from build123d import *

# Parameters (mm, degrees)
BOSS_EXTRUDE1_DEPTH     = 34
SKETCH2_R               = 35
BOSS_EXTRUDE2_DEPTH     = 10
SKETCH3_R               = 25
BOSS_EXTRUDE3_DEPTH     = 80
CUT_EXTRUDE2_START      = -40
CUT_EXTRUDE2_DEPTH      = 40
CUT_EXTRUDE5_DEPTH      = 114.247516529
CUT_EXTRUDE5_DEPTH_BACK = 114.247516529
SKETCH11_W              = 43
SKETCH11_H              = 18


with BuildPart() as part:
    # Sketch1 → Boss-Extrude1 (new body)
    with BuildSketch(Plane(origin=(0, 0, 0), x_dir=(1, 0, 0), z_dir=(0, 1, 0))):
        Polygon((50, 0), (-50, 0), (-50, 10), (-32.679491924, 40), (32.679491924, 40), (50, 10), align=None)
    extrude(amount=BOSS_EXTRUDE1_DEPTH)

    # Sketch2 → Boss-Extrude2 (add)
    with BuildSketch(Plane.XY):
        with Locations((0, 17)):
            Circle(SKETCH2_R)
    extrude(amount=-BOSS_EXTRUDE2_DEPTH)

    # Sketch3 → Boss-Extrude3 (add)
    with BuildSketch(Plane.XY):
        with Locations((0, 17)):
            Circle(SKETCH3_R)
    extrude(amount=-BOSS_EXTRUDE3_DEPTH)

    # Sketch5 → Cut-Extrude2 (cut)
    with BuildSketch(Plane(origin=(0, 0, -80), x_dir=(-1, 0, 0), z_dir=(0, 0, -1)).offset(CUT_EXTRUDE2_START)):
        with BuildLine():
            ThreePointArc((-25, 17.00000011), (-21.213203465, 3.771243492), (-11, -5.449944321))
            Line((-11, -5.449944321), (-11, 39.449944321))
            ThreePointArc((-11, 39.449944321), (-21.213203406, 30.228756602), (-25, 17.00000011))
        make_face()
        with BuildLine():
            ThreePointArc((-25, 17.00000011), (-21.213203406, 30.228756602), (-11, 39.449944321))
            Line((-11, 39.449944321), (-11, 52))
            Line((-11, 52), (-25, 52))
            Line((-25, 52), (-25, 17.00000011))
        make_face()
        with BuildLine():
            Line((-25, -18), (-11, -18))
            Line((-11, -18), (-11, -5.449944321))
            ThreePointArc((-11, -5.449944321), (-21.213203465, 3.771243492), (-25, 17.00000011))
            Line((-25, 17.00000011), (-25, -18))
        make_face()
        with BuildLine():
            ThreePointArc((25, 17), (21.213203436, 3.771243445), (11, -5.449944321))
            Line((11, -5.449944321), (11, -18))
            Line((11, -18), (25, -18))
            Line((25, -18), (25, 17))
        make_face()
        with BuildLine():
            Line((11, 39.449944321), (11, -5.449944321))
            ThreePointArc((11, -5.449944321), (21.213203436, 3.771243445), (25, 17))
            ThreePointArc((25, 17), (21.213203436, 30.228756555), (11, 39.449944321))
        make_face()
        with BuildLine():
            Line((11, 52), (11, 39.449944321))
            ThreePointArc((11, 39.449944321), (21.213203436, 30.228756555), (25, 17))
            Line((25, 17), (25, 52))
            Line((25, 52), (11, 52))
        make_face()
    extrude(amount=CUT_EXTRUDE2_DEPTH, mode=Mode.SUBTRACT)

    # Sketch11 → Cut-Extrude5 (cut, two sides: drawn at the far end of the back side and taken through both)
    with BuildSketch(Plane.ZY.offset(11).offset(-CUT_EXTRUDE5_DEPTH_BACK)):
        with Locations((-41.5, 17)):
            Rectangle(SKETCH11_W, SKETCH11_H)
    extrude(amount=CUT_EXTRUDE5_DEPTH + CUT_EXTRUDE5_DEPTH_BACK, mode=Mode.SUBTRACT)


solid = part.part
Geometry: final body of the model. Coordinates: model frame, mm. A direction names the side the tool comes from. Round coordinates to 2 decimals unless told otherwise and drop trailing zeros. Loops run counter-clockwise (first coordinate to the right, second up) from the corner with the lowest first, then second, coordinate; pieces in that order, holes last.
Q1. Pull-direction query (Z, two-part tool) for faces 5 (the flat face through (1, 8, -37)), 6 (the flat face through (-1, 17, 0)), 7 (the flat face through (0, 43, -10)), 8 (the flat face through (11, 17, -64)); classes: released by +Z, released by -Z, zero draft, split by the parting line, or undercut.
Q2. Material intervals for L1, parallel to Y at x = 11, z = -31; L2, parallel to Y at x = -29, z = -23; L3, parallel to Y at x = -36.5, z = -9.5, sorted ascending.
Q3. Section C-C on z = -5.5. Return loops of the section in (x, y), plus the area to 3 significant figures.
Q4. Access query for faces 1 (the flat face through (31, 34, -20)), 2 (the flat face through (1, 26, -37)), 3 (the flat face through (31, 0, -20)), 4 (the flat face through (-20, 31, -40)). Directions: +Z, -Z, +X, -X, +Y, -Y. A direction counts if a zero-diameter tool reaches every point of the face in a straight line with its end or side. Return the directions, or none.
Q5. Section B-B on y = 17. Return loops of the section in (x, z), plus the area to 3 significant figures.
Q6. Pin query (flat end, axial travel): P1, Ø3, axis at y = 13.5, z = -16.5, coming from the -X side; P2, Ø15, axis at x = -21.5, y = -2, coming from the -Z side; P3, Ø5, axis at y = 17.5, z = -14.5, coming from the +X side. Return the tip coordinate at first contact, or that it passes through.
Q7. Section D-D on x = 29. Return loops of the section in (y, z), plus the area to 3 significant figures.
Q8. Section A-A on z = -51.5. Return loops of the section in (x, y), plus the area to 3 significant figures.
Evaluation:
1. face 5: undercut
1. face 6: released by +Z
1. face 7: released by -Z
1. face 8: zero draft
2. L1: y = -5.45 to 8, 26 to 39.45
2. L2: y = 0 to 8, 26 to 34
2. L3: y = 0 to 34
3. outline: (-50, 0) - (-30.59, 0) arc R35 ccw to (30.59, 0) - (50, 0) - (50, 34) - (30.59, 34) arc R35 ccw to (-30.59, 34) - (-50, 34) - close
3. area: 4,970 mm2
4. face 1: -Z, +X, +Y
4. face 2: +X, -X
4. face 3: -Z, +X, -Y
4. face 4: -Z, -X, +Y, -Y
5. outline: (-50, -10) - (-44.23, -20) - (44.23, -20) - (50, -10) - (50, 0) - (-50, 0) - close; (-11, -80) - (11, -80) - (11, -63) - (-11, -63) - close
5. area: 2,320 mm2
6. P1: stops at x = -47.11
6. P2: stops at z = -40
6. P3: stops at x = 48.85
7. outline: (-2.6, -10) - (0, -10) - (0, -40) - (8, -40) - (8, -20) - (26, -20) - (26, -40) - (34, -40) - (34, -10) - (36.6, -10) - (36.6, 0) - (-2.6, 0) - close
7. area: 1,050 mm2
8. outline: (-11, -5.45) arc R25 ccw to (11, -5.45) - (11, 8) - (-11, 8) - close; (-11, 26) - (11, 26) - (11, 39.45) arc R25 ccw to (-11, 39.45) - close
8. area: 667 mm2
